CAD build for the part. Positions are in the model's coordinates, mm. A direction names the side the tool comes from. Round coordinates to 2 decimals unless told otherwise and drop trailing zeros. Loops run counter-clockwise (first coordinate to the right, second up) from the corner with the lowest first, then second, coordinate; pieces in that order, holes last. Notation, with made-up numbers: M 3,84.25 L 13,84.25 A15 cw 13,107.25 Z; hole C -3,72.5 d1. An arc over 180 degrees is marked long. One line per item, written item: value. Start each with the question number.
from build123d import *

# Parameters (mm, degrees)
F1_DEPTH = 19.05
F2_DEPTH = 114.3
F3_W     = 114.3
F3_H     = 101.6
F4_DEPTH = 177.8


with BuildPart() as f1:
    # F0 (on Right) → F1 (new body)
    with BuildSketch(Plane.YZ):
        with BuildLine():
            Line((-50.8, 0), (50.8, 0))
            ThreePointArc((50.8, 0), (0, 50.8), (-50.8, 0))
        make_face()
        with BuildLine():
            Line((50.8, -101.6), (50.8, 0))
            ThreePointArc((50.8, 0), (0, -50.8), (-50.8, 0))
            Line((-50.8, 0), (-50.8, -101.6))
            Line((-50.8, -101.6), (50.8, -101.6))
        make_face()
        with BuildLine():
            ThreePointArc((-50.8, 0), (0, -50.8), (50.8, 0))
            Line((50.8, 0), (-50.8, 0))
        make_face()
    extrude(amount=F1_DEPTH)

    # F0 (on Right) → F2 (join)
    with BuildSketch(Plane.YZ):
        with BuildLine():
            Line((50.8, -101.6), (50.8, 0))
            ThreePointArc((50.8, 0), (0, -50.8), (-50.8, 0))
            Line((-50.8, 0), (-50.8, -101.6))
            Line((-50.8, -101.6), (50.8, -101.6))
        make_face()
    extrude(amount=F2_DEPTH)

    # F3 (on face) → F4 (join)
    with BuildSketch(Plane(origin=(0, 0, -101.6), x_dir=(1, 0, 0), z_dir=(0, 0, -1))):
        with Locations((57.15, 0)):
            Rectangle(F3_W, F3_H)
    extrude(amount=F4_DEPTH)


solid = f1.part
(1) Slice it at B-B, the plane x = 81.5. List the corners of the cut face in (y, z).
(2) Which spindle directions (+Z, -Z, +X, -X, +Y, -Y) get a long thin tool onto all of the face, cutting with end or side? Do faces 1 (the flat face through (19.05, -1, 1)), 2 (the flat face through (56, 50.8, -138)). Say none if no direction does.
(3) Slice it at A-A, the plane y = 0. List the corners of the cut face in (x, z), and give its area (3 significant figures).
(4) Probe L1, parallel to X at y = -28, z = -7.5; L2, parallel to Y at x = 88.5, z = -6; L3, parallel to Y at x = 99.5, z = -12. List the from-to ranges inside material, lowest first.
(5) Slice it at C-C, the plane y = 32. List the corners of the cut face in (x, z).
(6) Mould opens along Y. For faces 3 (the flat face through (0, 1, -112)), 4 (the cylindrical face through (66.008, 1.117, -50.788)), 5 (the cylindrical face through (9.392, 1.117, 50.788)) say: pulls with the +Y half, pulls with the -Y half, needs draft (parallel to the pull), parting line crosses it, or undercut.
Check result:
1. outline: M -50.8,-279.4 L 50.8,-279.4 L 50.8,0 A50.8 cw -50.8,0 Z
2. face 1: +Z, +X
2. face 2: +Z, -Z, +X, -X, +Y
3. outline: M 0,-279.4 L 114.3,-279.4 L 114.3,-50.8 L 19.05,-50.8 L 19.05,50.8 L 0,50.8 Z
3. area: 28,100 mm^2
4. L1: x = 0 to 19.05
4. L2: y = -50.8 to -50.44, 50.44 to 50.8
4. L3: y = -50.8 to -49.36, 49.36 to 50.8
5. outline: M 0,-279.4 L 114.3,-279.4 L 114.3,-39.45 L 19.05,-39.45 L 19.05,39.45 L 0,39.45 Z
6. face 3: needs draft
6. face 4: undercut
6. face 5: parting line crosses it
